Autodesk Inventor part; units mm, degrees
ref_plane "YZ Plane" through (0, 0, 0) normal (1, 0, 0) x (0, 1, 0)
ref_plane "XZ Plane" through (0, 0, 0) normal (0, 1, 0) x (-1, 0, 0)
ref_plane "XY Plane" through (0, 0, 0) normal (0, 0, 1) x (1, 0, 0)
sketch "Sketch1" plane through (0, 0, 0) normal (0, 1, 0) x (-1, 0, 0)
  circle A0 centre (0, 0) radius 11
  dimension "d0" = 22
extrude "Extrusion1" add sketch "Sketch1" along normal blind 2
sketch "Sketch2" plane through (0, 2, 0) normal (0, 1, 0) x (1, 0, 0)
  circle A0 centre (0, 0) radius 11
  circle A1 centre (0, 0) radius 9.25
  dimension "d3" = 18.5
extrude "Extrusion2" add sketch "Sketch2" along normal blind 6.5 contours A1
fillet "Fillet1" radius 2 1 edges at (-9.25, 8.5, 0)
sketch "Sketch3" plane through (0, 0, 0) normal (0, -1, 0) x (1, 0, 0)
  circle A0 centre (0, 0) radius 11
  circle A1 centre (0, 0) radius 12
  dimension "d7" = 24
extrude "Extrusion3" add sketch "Sketch3" along normal blind 2 contours A0 | A1
chamfer "Chamfer1" distance 0.5 angle 45 1 edges at (11, 2, 0)
sketch "Sketch4" plane through (0, -2, 0) normal (0, -1, 0) x (1, 0, 0)
  circle A0 centre (0, 0) radius 12
  circle A1 centre (0, 0) radius 5
  dimension "d13" = 10
extrude "Extrusion4" cut sketch "Sketch4" against normal blind 10 contours A1
sketch "Sketch5" plane through (0, -2, 0) normal (0, -1, 0) x (1, 0, 0)
  circle A0 centre (0, 0) radius 5
  circle A1 centre (0, 0) radius 12
  circle A2 centre (0, 0) radius 6.2
  dimension "d16" = 12.4
extrude "Extrusion5" cut sketch "Sketch5" against normal blind 2 contours A2
properties part number "guzik"
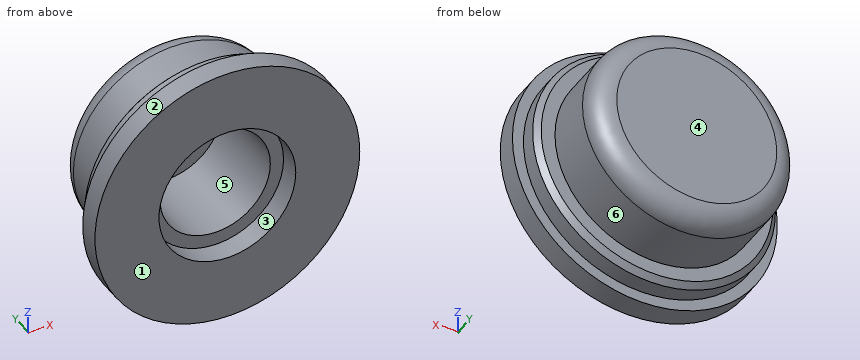
Part model, mm, in its own coordinate system. Face numbers are marked on the shaded views. A direction names the side the tool comes from. Coordinates: 2 decimals unless noted, no trailing zeros. Loops run counter-clockwise (first coordinate to the right, second up) from the corner with the lowest first, then second, coordinate; pieces in that order, holes last. Notation, with made-up numbers: (46, 26) - (69, 26) arc R25 ccw to (69, 64) - close; hole circle Ø2 at (78, 84.5). An arc over 180 degrees is marked (long way). Write item = value, one per line. Start each with the question number.
Item 1: 3-axis set-ups, long thin cutter, end or side, ignore diameter. For the marked faces 4, 5 and 6: which of +Z, -Z, +X, -X, +Y, -Y reach the whole face in a straight line?
Item 2: Mould opens along Z. For the marked faces 1, 2 and 3 say: released by +Z, released by -Z, zero draft, split by the parting line, or undercut.
Item 3: Wall check: L1, parallel to Z at x = 0, y = -0.6; L2, parallel to Y at x = -3.5, z = 3.25; L3, parallel to Y at x = 2, z = 9.75. Give the ranges that are in metal, low to high. Write a range as from..to.
Item 4: Cut at C-C, the plane y = 3. Give the cut face in (x, z).
Item 5: Flat gauge pins, fed straight in: pin 1 Ø2 at (x, y) = (0.5, 3.5) entering from -Z; pin 2 Ø3.5 at (x, z) = (0.5, 1) entering from -Y; pin 3 Ø1.5 at (x, z) = (-4.5, 0) entering from -Y. Where does each tip first touch, or does it go through?
Item 6: Cut at A-A, the plane x = 0. Give the cut face in (y, z).
Item 7: Cut at D-D, the plane y = -1. Give the cut face in (x, z).
Item 8: Cut at B-B, the plane z = 0. Give the cut face in (x, y), and give its area (3 significant figures).
The answers:
q1.face_4 = +Z, -Z, +X, -X, +Y
q1.face_5 = -Y
q1.face_6 = +Y
q2.face_1 = zero draft
q2.face_2 = split by the parting line
q2.face_3 = undercut
q3.L1 = -12..-6.2, 6.2..12
q3.L2 = 8..8.5
q3.L3 = -2..2
q4.outline = circle Ø18.5 at (0, 0); hole circle Ø10 at (0, 0)
q5.pin_1 = -9.25
q5.pin_2 = 8
q5.pin_3 = 0
q6.outline = (-2, -12) - (0, -12) - (0, -11) - (1.5, -11) - (2, -10.5) - (2, -9.25) - (6.5, -9.25) arc R2 ccw to (8.5, -7.25) - (8.5, 7.25) arc R2 ccw to (6.5, 9.25) - (2, 9.25) - (2, 10.5) - (1.5, 11) - (0, 11) - (0, 12) - (-2, 12) - (-2, 6.2) - (0, 6.2) - (0, 5) - (8, 5) - (8, -5) - (0, -5) - (0, -6.2) - (-2, -6.2) - close
q7.outline = circle Ø24 at (0, 0); hole circle Ø12.4 at (0, 0)
q8.outline = (-12, -2) - (-6.2, -2) - (-6.2, 0) - (-5, 0) - (-5, 8) - (5, 8) - (5, 0) - (6.2, 0) - (6.2, -2) - (12, -2) - (12, 0) - (11, 0) - (11, 1.5) - (10.5, 2) - (9.25, 2) - (9.25, 6.5) arc R2 ccw to (7.25, 8.5) - (-7.25, 8.5) arc R2 ccw to (-9.25, 6.5) - (-9.25, 2) - (-10.5, 2) - (-11, 1.5) - (-11, 0) - (-12, 0) - close
q8.area = 105 mm2
